Input: part model. Units: mm. Frame: model coordinates. Give positions to 0.01 mm unless a question says otherwise; leave off trailing zeros. Loops run counter-clockwise (first coordinate to the right, second up) from the corner with the lowest first, then second, coordinate; pieces in that order, holes last.
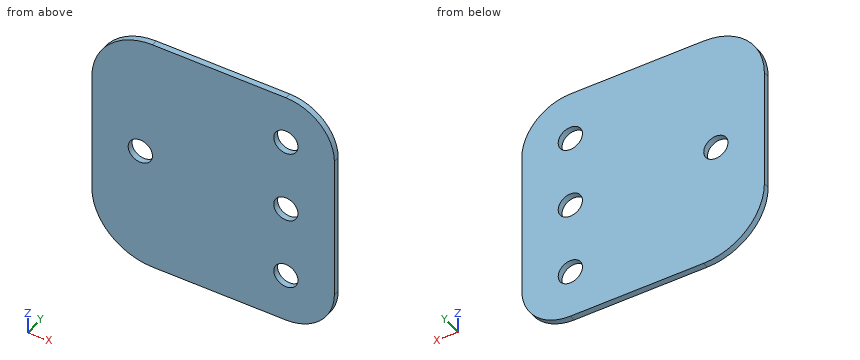
from build123d import *

# Parameters (mm, degrees)
SKETCH1_R           = 3.175
BOSS_EXTRUDE1_DEPTH = 1.5875


with BuildPart() as part:
    # Sketch1 → Boss-Extrude1 (new body)
    with BuildSketch(Plane(origin=(0, 0, 0), x_dir=(1, 0, 0), z_dir=(0, 1, 0))):
        with BuildLine():
            Line((-47.625, 0), (-12.7, 0))
            ThreePointArc((-12.7, 0), (-3.719743879, 3.719743879), (0, 12.7))
            Line((0, 12.7), (0, 50.8))
            ThreePointArc((0, 50.8), (-3.719743879, 59.780256121), (-12.7, 63.5))
            Line((-12.7, 63.5), (-47.625, 63.5))
            ThreePointArc((-47.625, 63.5), (-58.850320151, 58.850320151), (-63.5, 47.625))
            Line((-63.5, 47.625), (-63.5, 44.45))
            Line((-63.5, 44.45), (-63.5, 19.05))
            Line((-63.5, 19.05), (-63.5, 15.875))
            ThreePointArc((-63.5, 15.875), (-58.850320151, 4.649679849), (-47.625, 0))
        make_face()
        with Locations((-12.7, 12.7)):
            Circle(SKETCH1_R, mode=Mode.SUBTRACT)
        with Locations((-50.8, 31.75)):
            Circle(SKETCH1_R, mode=Mode.SUBTRACT)
        with Locations((-12.7, 31.75)):
            Circle(SKETCH1_R, mode=Mode.SUBTRACT)
        with Locations((-12.7, 50.8)):
            Circle(SKETCH1_R, mode=Mode.SUBTRACT)
    extrude(amount=BOSS_EXTRUDE1_DEPTH)


solid = part.part
(1) Cut plane D-D (z = -13.5). Return the cut outline in (x, y), and give its area (3 significant figures).
Values follow:
outline: (-63.32, 0) - (-15.77, 0) - (-15.77, 1.59) - (-63.32, 1.59) - close; (-9.63, 0) - (0, 0) - (0, 1.59) - (-9.63, 1.59) - close
area: 90.8 mm2
(2) Cut plane C-C (y = 1.1). Return the cut outline in (x, z) (3 decimals), and give its area (3 significant figures).
Values follow:
outline: (-63.5, -47.625) arc R15.875 ccw to (-47.625, -63.5) - (-12.7, -63.5) arc R12.7 ccw to (0, -50.8) - (0, -12.7) arc R12.7 ccw to (-12.7, 0) - (-47.625, 0) arc R15.875 ccw to (-63.5, -15.875) - close; hole circle Ø6.35 at (-50.8, -31.75); hole circle Ø6.35 at (-12.7, -50.8); hole circle Ø6.35 at (-12.7, -31.75); hole circle Ø6.35 at (-12.7, -12.7)
area: 3,730 mm2
(3) Cut plane B-B (x = -50.8). Return the cut outline in (y, z) (1 decimal), and give its area (3 significant figures).
Values follow:
outline: (0, -63.2) - (1.6, -63.2) - (1.6, -34.9) - (0, -34.9) - close; (0, -28.6) - (1.6, -28.6) - (1.6, -0.3) - (0, -0.3) - close
area: 89.7 mm2
(4) Cut plane A-A (z = -31.75). Return the cut outline in (x, y) (1 decimal).
Values follow:
outline: (-63.5, 0) - (-54, 0) - (-54, 1.6) - (-63.5, 1.6) - close; (-47.6, 0) - (-15.9, 0) - (-15.9, 1.6) - (-47.6, 1.6) - close; (-9.5, 0) - (0, 0) - (0, 1.6) - (-9.5, 1.6) - close
(5) Ray query, probe 1 along Z at (x, y) = (-12.7, 0.65) (3 decimals); probe 2 along X at (y, z) = (1.4, -32); probe 3 along Z at (x, y) = (-51.5, 0.4). Return the intervals inside material, ascending.
Values follow:
probe 1: z = -63.5 to -53.975, -47.625 to -34.925, -28.575 to -15.875, -9.525 to 0
probe 2: x = -63.5 to -53.97, -47.63 to -15.87, -9.53 to 0
probe 3: z = -63.02 to -34.85, -28.65 to -0.48
